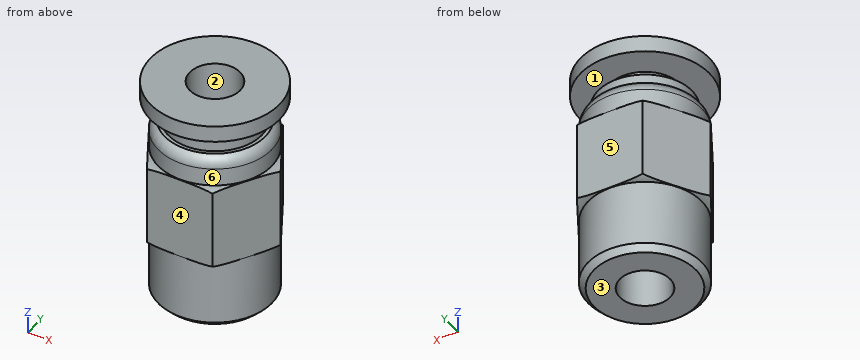
from build123d import *

# Parameters (mm, degrees)
F2_R     = 2.15
F3_DEPTH = 19.001
F4_R     = 9
F5_DEPTH = 14
F6_SIZE  = 0.5


with BuildPart() as f1:
    # F0 (on Front) → F1 (revolve)
    with BuildSketch(Plane.XZ):
        with BuildLine():
            Line((0, 19), (0, 0))
            Line((0, 0), (4.85, 0))
            Line((4.85, 0), (4.85, 6.1))
            ThreePointArc((4.85, 6.1), (6.160773, 6.512059), (7, 7.6))
            Line((7, 7.6), (7, 11.6))
            ThreePointArc((7, 11.6), (6.160773, 12.687941), (4.85, 13.1))
            Line((4.85, 13.1), (4.85, 14.6))
            ThreePointArc((4.85, 14.6), (4.703428, 15.170636), (4.3, 15.6))
            Line((4.3, 15.6), (4, 15.6))
            Line((4, 15.6), (4, 16.6))
            Line((4, 16.6), (3, 16.6))
            Line((3, 16.6), (3, 17.6))
            Line((3, 17.6), (5.5, 17.6))
            Line((5.5, 17.6), (5.5, 19))
            Line((5.5, 19), (0, 19))
        make_face()
    revolve(axis=Axis((0, 0, 9.5), (0, 0, 1)))

    # F2 (on face) → F3 (cut, through all)
    with BuildSketch(Plane.XY.offset(19)):
        Circle(F2_R)
    extrude(amount=-F3_DEPTH, mode=Mode.SUBTRACT)

    # F4 (on face) → F5 (cut)
    with BuildSketch(Plane(origin=(0, 0, 0), x_dir=(1, 0, 0), z_dir=(0, 0, -1))):
        Circle(F4_R)
        Polygon((-2.829016, 4.9), (2.829016, 4.9), (5.658033, 0), (2.829016, -4.9), (-2.829016, -4.9), (-5.658033, 0), align=None, mode=Mode.SUBTRACT)
    extrude(amount=-F5_DEPTH, mode=Mode.SUBTRACT)

    # F6
    f6_edges = [f1.edges().sort_by_distance(p)[0] for p in [
        (-4.85, 0, 0),
    ]]
    chamfer(f6_edges, length=F6_SIZE)


solid = f1.part
Could you check a few things on this model? Use its own coordinates, in mm. Face numbers are marked on the shaded views. A direction names the side the tool comes from. Round coordinates to 2 decimals unless told otherwise and drop trailing zeros. Order: outer loops, then holes, each group sorted by start corner. A loop starts at its lowest first (then second) coordinate and runs counter-clockwise, first axis right, second up.
(1) Please list where these lines run through material, in increasing order: line 1 along Z through (x, y) = (-0.75, 4); line 2 along Y through (x, z) = (0, 11); line 3 along Z through (x, y) = (-1.5, -2.75).
Response values:
line 1: z = 0 to 15.6, 17.6 to 19
line 2: y = -4.9 to -2.15, 2.15 to 4.9
line 3: z = 0 to 16.6, 17.6 to 19
(2) I'm going to push flat-ended pins straight in: pin 1 (1 mm diameter, centred on x = 3.5, z = 6, fed in from +Y); pin 2 (3 mm diameter, centred on y = -2.5, z = 12, fed in from -X); pin 3 (4.5 mm diameter, centred on x = 0, z = 10, fed in from +Y). Where does each tip first touch, or does it pass through?
Response values:
pin 1: stops at y = 4.54
pin 2: stops at x = -5.08
pin 3: stops at y = 4.9
(3) If we mould it in two halves opening along Z, with no side actions, what happens to the marked faces 1, 2 and 3? For each: released by +Z, released by -Z, zero draft, split by the parting line, or undercut.
Response values:
face 1: undercut
face 2: zero draft
face 3: released by -Z
(4) Which directions (+Z, -Z, +X, -X, +Y, -Y) give clear straight access to the entire face, cutting with the end or side of a thin tool? Please do the marked faces 4, 5 and 6.
Response values:
face 4: -Z, +X, -X, -Y
face 5: -Z, +X, -X, +Y
face 6: none
(5) Imagine slicing it at C-C (z = 17). Write out the boundary of the cut face in (x, y), plus the area to 3 significant figures.
Response values:
outline: circle Ø6 at (0, 0); hole circle Ø4.3 at (0, 0)
area: 13.8 mm2
(6) Imagine slicing it at B-B (z = 3). Write out the boundary of the cut face in (x, y).
Response values:
outline: circle Ø9.7 at (0, 0); hole circle Ø4.3 at (0, 0)
